Job drawing, mm, ordinate dimensions from the low corner. One solid piece. Round coordinates to 2 decimals unless told otherwise and drop trailing zeros. Write each loop counter-clockwise with the first axis right and the second up, starting at its lowest first coordinate (ties: lowest second). Pieces come first, ordered by that corner, then holes.
1) Flat gauge pin, fed straight in: pin 1 (0.5 mm diameter, centred on y = 0.5, z = 7, fed in from +X). Where does the tip first touch, or does it go through?
2) Saw through at C-C on y = 0.7. Write the cut outline in (x, z), and give its area (3 significant figures).
3) Saw through at D-D on z = 14.5. Write the cut outline in (x, y), and give its area (3 significant figures).
4) Saw through at A-A on z = 7.38. Write the cut outline in (x, y).
5) Drill centre lines: L1, parallel to X at y = 0.7, z = 7.38; L2, parallel to Z at x = 6, y = 0.35; L3, parallel to Z at x = 45, y = 0.75. Where is each one in solid material? Low to high.
6) Saw through at B-B on x = 17.05. Write the cut outline in (y, z), and give its area (3 significant figures).
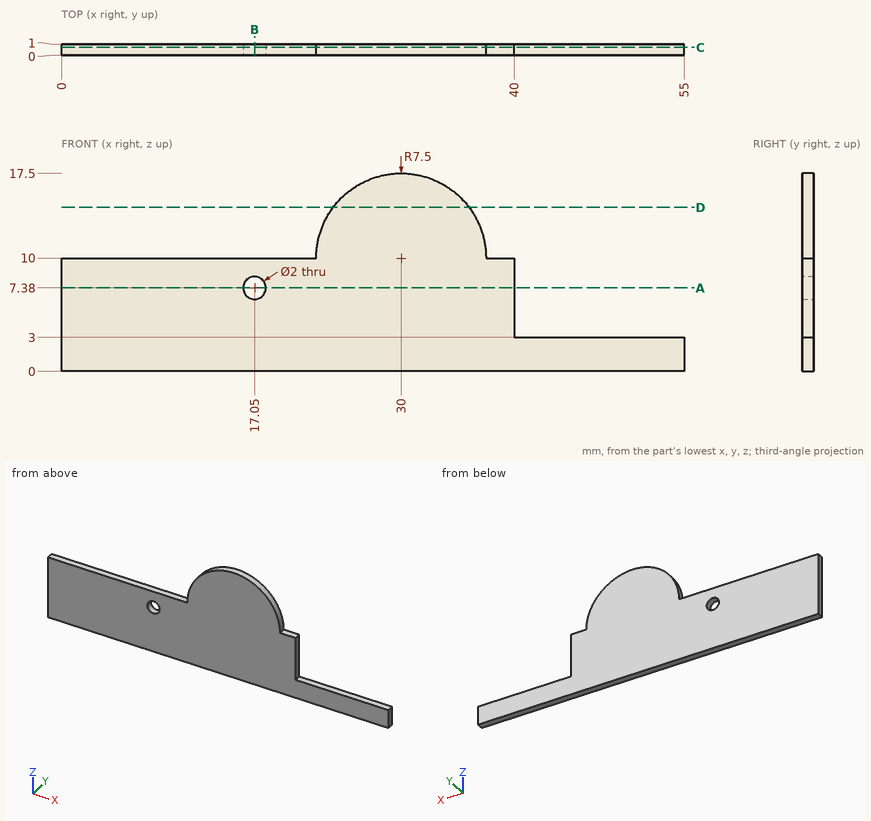
Completed:
1. pin 1: stops at x = 40
2. outline: (0, 0) - (55, 0) - (55, 3) - (40, 3) - (40, 10) - (37.5, 10) arc R7.5 ccw to (22.5, 10) - (0, 10) - close; hole circle Ø2 at (17.05, 7.38)
2. area: 530 mm2
3. outline: (24, 0) - (36, 0) - (36, 1) - (24, 1) - close
3. area: 12.0 mm2
4. outline: (0, 0) - (16.05, 0) - (16.05, 1) - (0, 1) - close; (18.05, 0) - (40, 0) - (40, 1) - (18.05, 1) - close
5. L1: x = 0 to 16.05, 18.05 to 40
5. L2: z = 0 to 10
5. L3: z = 0 to 3
6. outline: (0, 0) - (1, 0) - (1, 6.38) - (0, 6.38) - close; (0, 8.38) - (1, 8.38) - (1, 10) - (0, 10) - close
6. area: 8.00 mm2
